Here's how the part is built. I have some questions about the finished solid (model axes, mm). Face numbers are marked on the shaded views. A direction names the side the tool comes from. Round coordinates to 2 decimals unless told otherwise and drop trailing zeros. Order: outer loops, then holes, each group sorted by start corner. A loop starts at its lowest first (then second) coordinate and runs counter-clockwise, first axis right, second up. Notation, with made-up numbers: (-32, 86) -> (-20, 86) arc R16 ccw to (-20, 90) -> close; hole circle Ø3 at (36.5, -11). An arc over 180 degrees is marked (long way). Use a Markdown table: item, result. Add a question column.
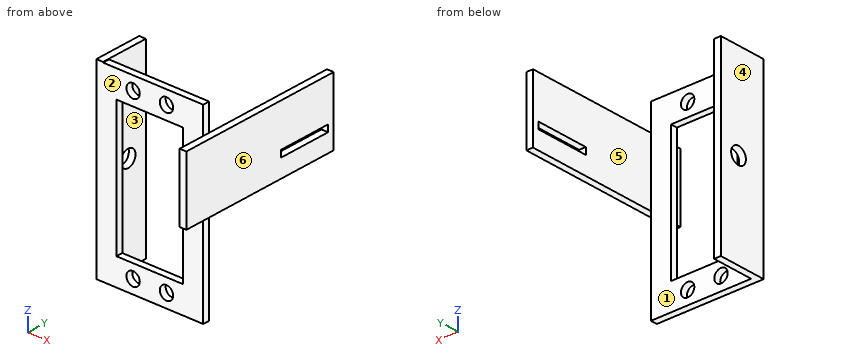
from build123d import *

# Parameters (mm, degrees)
SKETCH1_W             = 20
SKETCH1_H             = 8
SKETCH1_R             = 2
BOSS_EXTRUDE1_DEPTH   = 2
BOSS_EXTRUDE1_2_DEPTH = 2
SKETCH6_W             = 56
SKETCH6_H             = 2
BOSS_EXTRUDE5_DEPTH   = 6
SKETCH10_W            = 56
SKETCH10_H            = 2
BOSS_EXTRUDE7_DEPTH   = 4
SKETCH11_W            = 56.175194469
SKETCH11_H            = 14.528307745
BOSS_EXTRUDE8_DEPTH   = 2
SKETCH12_R            = 2.5
CUT_EXTRUDE3_DEPTH    = 2
SKETCH13_W            = 20
SKETCH13_H            = 50
SKETCH13_W_2          = 2
SKETCH13_H_2          = 16
BOSS_EXTRUDE9_DEPTH   = 2


with BuildPart() as part:
    # Sketch1 → Boss-Extrude1 (new body)
    with BuildSketch(Plane(origin=(0, 0, 0), x_dir=(1, 0, 0), z_dir=(0, 1, 0))):
        with Locations((-0.385906166, -15.501316712)):
            Rectangle(SKETCH1_W, SKETCH1_H)
        with Locations(Location((4.614093834, -15.501316712, 0), (0, 0, 270))):
            Circle(SKETCH1_R, mode=Mode.SUBTRACT)
        with Locations(Location((-5.385906166, -15.501316712, 0), (0, 0, 270))):
            Circle(SKETCH1_R, mode=Mode.SUBTRACT)
    extrude(amount=BOSS_EXTRUDE1_DEPTH)



with BuildPart() as body_2:
    # Sketch1 → Boss-Extrude1 2 (new body)
    with BuildSketch(Plane(origin=(0, 0, 0), x_dir=(1, 0, 0), z_dir=(0, 1, 0))):
        with Locations((-0.385906166, 32.498683288)):
            Rectangle(SKETCH1_W, SKETCH1_H)
        with Locations(Location((4.614093834, 32.498683288, 0), (0, 0, 270))):
            Circle(SKETCH1_R, mode=Mode.SUBTRACT)
        with Locations(Location((-5.385906166, 32.498683288, 0), (0, 0, 270))):
            Circle(SKETCH1_R, mode=Mode.SUBTRACT)
    extrude(amount=BOSS_EXTRUDE1_2_DEPTH)


with BuildPart() as part_1:
    add(part.part)

    add(body_2.part)  # Boss-Extrude5 merges body 2
    # Sketch6 → Boss-Extrude5 (add)
    with BuildSketch(Plane(origin=(9.614093834, 0, 0), x_dir=(0, 0, -1), z_dir=(1, 0, 0))):
        with Locations((8.498683288, 1)):
            Rectangle(SKETCH6_W, SKETCH6_H)
    extrude(amount=BOSS_EXTRUDE5_DEPTH)

    # Sketch10 → Boss-Extrude7 (add)
    with BuildSketch(Plane.ZY.offset(10.385906166)):
        with Locations((-8.498683288, 1)):
            Rectangle(SKETCH10_W, SKETCH10_H)
    extrude(amount=BOSS_EXTRUDE7_DEPTH)

    # Sketch11 → Boss-Extrude8 (add)
    with BuildSketch(Plane.ZY.offset(14.385906166)):
        with Locations((-8.411086054, 7.264153873)):
            Rectangle(SKETCH11_W, SKETCH11_H)
    extrude(amount=BOSS_EXTRUDE8_DEPTH)

    # Sketch12 → Cut-Extrude3 (cut)
    with BuildSketch(Plane.ZY.offset(16.385906166)):
        with Locations((-8.411086053, 8.528307745)):
            Circle(SKETCH12_R)
    extrude(amount=-CUT_EXTRUDE3_DEPTH, mode=Mode.SUBTRACT)

    # Sketch13 → Boss-Extrude9 (add)
    with BuildSketch(Plane(origin=(15.614093834, 0, 0), x_dir=(0, 0, -1), z_dir=(1, 0, 0))):
        with Locations((-1.501316712, 17)):
            Rectangle(SKETCH13_W, SKETCH13_H)
        with Locations((2.10225409, 32.102958265)):
            Rectangle(SKETCH13_W_2, SKETCH13_H_2, mode=Mode.SUBTRACT)
    extrude(amount=BOSS_EXTRUDE9_DEPTH)


solid = part_1.part
(1) Please list where these lines run through material, in increasing order: probe 1 along X at (y, z) = (3, -6.5); probe 2 along X at (y, z) = (8, -26.5); probe 3 along X at (y, z) = (16.5, 3). Write a range as from..to.
(2) I want a section at B-B on z = -22.5. List the corners of the cut face in (x, y) for me.
(3) I want a section at C-C on x = -0.5. List the corners of the cut face in (y, z) for me, and give its area (3 significant figures).
(4) I want a section at A-A on y = 4. List the corners of the cut face in (x, z) for me, and give its area (3 significant figures).
(5) If we mould it in two halves opening along X, with no side actions, what happens to the marked faces 1, 2, 3 and 4? For each: pulls with the +X half, pulls with the -X half, needs draft (parallel to the pull), parting line crosses it, or undercut.
(6) I want a section at D-D on y = 9.5. List the corners of the cut face in (x, z) for me, and give its area (3 significant figures).
(7) On a 3-axis mill with a long thin cutter (end or side, diameter ignored), from which of +Z, -Z, +X, -X, +Y, -Y can I reach the whole of each face in a straight line? I mean the marked faces 5 and 6. Say none if no direction works.
(8) I'm going to push flat-ended pins straight in: P1, Ø1, axis at y = 0.5, z = -17.5, coming from the +X side; P2, Ø5, axis at x = 4.61, z = 15.5, coming from the +Y side; P3, Ø12, axis at y = 29.5, z = -10.5, coming from the -X side. Where does each tip first touch, or does it pass through?
Output:
| question | item | result |
|---|---|---|
| 1 | probe 1 | -16.39..-14.39, 15.61..17.61 |
| 1 | probe 2 | -16.39..-14.39 |
| 1 | probe 3 | 15.61..17.61 |
| 2 | outline | (-16.39, 0) -> (-10.39, 0) -> (-10.39, 2) -> (-14.39, 2) -> (-14.39, 14.53) -> (-16.39, 14.53) -> close; (9.61, 0) -> (15.61, 0) -> (15.61, 2) -> (9.61, 2) -> close |
| 3 | outline | (0, -36.5) -> (2, -36.5) -> (2, -28.5) -> (0, -28.5) -> close; (0, 11.5) -> (2, 11.5) -> (2, 19.5) -> (0, 19.5) -> close |
| 3 | area | 32.0 mm² |
| 4 | outline | (-16.39, -36.5) -> (-14.39, -36.5) -> (-14.39, 19.68) -> (-16.39, 19.68) -> close; (15.61, -8.5) -> (17.61, -8.5) -> (17.61, 11.5) -> (15.61, 11.5) -> close |
| 4 | area | 152 mm² |
| 5 | face 1 | undercut |
| 5 | face 2 | needs draft |
| 5 | face 3 | undercut |
| 5 | face 4 | pulls with the -X half |
| 6 | outline | (-16.39, -36.5) -> (-14.39, -36.5) -> (-14.39, -10.71) -> (-16.39, -10.71) -> close; (-16.39, -6.11) -> (-14.39, -6.11) -> (-14.39, 19.68) -> (-16.39, 19.68) -> close; (15.61, -8.5) -> (17.61, -8.5) -> (17.61, 11.5) -> (15.61, 11.5) -> close |
| 6 | area | 143 mm² |
| 7 | face 5 | +Z, -Z, +Y |
| 7 | face 6 | +Z, -Z, +X, +Y, -Y |
| 8 | P1 | x = 15.61 |
| 8 | P2 | y = 2 |
| 8 | P3 | x = 15.61 |
